```python
from build123d import *

# Parameters (mm, degrees)
SKETCH1_W           = 47.5
SKETCH1_H           = 38.5
SKETCH1_R           = 6.25
SKETCH1_R_2         = 2.75
BOSS_EXTRUDE2_DEPTH = 1
SKETCH2_W           = 61.5
SKETCH2_H           = 44.5
SKETCH2_R           = 1.55
SKETCH2_W_2         = 47.5
SKETCH2_H_2         = 38.5
BOSS_EXTRUDE3_DEPTH = 11.3
SKETCH3_R           = 1.55
BOSS_EXTRUDE4_DEPTH = 2
FILLET2_R           = 4
SKETCH4_W           = 16
SKETCH4_H           = 5.5
CUT_EXTRUDE1_DEPTH  = 8


with BuildPart() as part:
    # Sketch1 → Boss-Extrude2 (new body)
    with BuildSketch(Plane(origin=(0, 0, 0), x_dir=(1, 0, 0), z_dir=(0, 1, 0))):
        Rectangle(SKETCH1_W, SKETCH1_H)
        with Locations(Location((-2.25, 9.8, 0), (0, 0, 270))):
            Circle(SKETCH1_R, mode=Mode.SUBTRACT)
        with Locations(Location((10.75, 0, 0), (0, 0, 270))):
            Circle(SKETCH1_R, mode=Mode.SUBTRACT)
        with Locations(Location((-15.25, 0, 0), (0, 0, 270))):
            Circle(SKETCH1_R, mode=Mode.SUBTRACT)
        with Locations(Location((-2.25, -9.8, 0), (0, 0, 270))):
            Circle(SKETCH1_R, mode=Mode.SUBTRACT)
        with Locations(Location((11.75, 12.05, 0), (0, 0, 270))):
            Circle(SKETCH1_R_2, mode=Mode.SUBTRACT)
    extrude(amount=BOSS_EXTRUDE2_DEPTH)

    # Sketch2 → Boss-Extrude3 (add)
    with BuildSketch(Plane(origin=(0, 1, 0), x_dir=(1, 0, 0), z_dir=(0, 1, 0))):
        Rectangle(SKETCH2_W, SKETCH2_H)
        with Locations(Location((-27.25, 18.75, 0), (0, 0, 270))):
            Circle(SKETCH2_R, mode=Mode.SUBTRACT)
        with Locations(Location((27.25, 18.75, 0), (0, 0, 90))):
            Circle(SKETCH2_R, mode=Mode.SUBTRACT)
        with Locations(Location((27.25, -18.75, 0), (0, 0, 270))):
            Circle(SKETCH2_R, mode=Mode.SUBTRACT)
        with Locations(Location((-27.25, -18.75, 0), (0, 0, 90))):
            Circle(SKETCH2_R, mode=Mode.SUBTRACT)
        Rectangle(SKETCH2_W_2, SKETCH2_H_2, mode=Mode.SUBTRACT)
    extrude(amount=-BOSS_EXTRUDE3_DEPTH)

    # Sketch3 → Boss-Extrude4 (add)
    with BuildSketch(Plane.XZ.offset(-1)):
        with Locations(Location((27.25, -18.75, 0), (0, 0, 270))):
            Circle(SKETCH3_R)
        with Locations(Location((27.25, 18.75, 0), (0, 0, 90))):
            Circle(SKETCH3_R)
        with Locations(Location((-27.25, 18.75, 0), (0, 0, 270))):
            Circle(SKETCH3_R)
        with Locations(Location((-27.25, -18.75, 0), (0, 0, 90))):
            Circle(SKETCH3_R)
    extrude(amount=BOSS_EXTRUDE4_DEPTH)

    # Fillet2
    fillet2_edges = [part.edges().sort_by_distance(p)[0] for p in [
        (-30.75, -4.65, 22.25),
        (-30.75, -4.65, -22.25),
        (30.75, -4.65, -22.25),
        (30.75, -4.65, 22.25),
    ]]
    fillet(fillet2_edges, radius=FILLET2_R)

    # Sketch4 → Cut-Extrude1 (cut)
    with BuildSketch(Plane.ZY.offset(-23.75)):
        with Locations((-5.75, -7.55)):
            Rectangle(SKETCH4_W, SKETCH4_H)
    extrude(amount=-CUT_EXTRUDE1_DEPTH, mode=Mode.SUBTRACT)


solid = part.part
```
Geometry: final body of the model. Coordinates: model frame, mm. A direction names the side the tool comes from. Coordinates: 2 decimals unless noted, no trailing zeros. Loops run counter-clockwise (first coordinate to the right, second up) from the corner with the lowest first, then second, coordinate; pieces in that order, holes last. Notation, with made-up numbers: (22, -8.75) -> (50, -8.75) arc R20 ccw to (50, 2.25) -> close; hole circle Ø4 at (59, -13). An arc over 180 degrees is marked (long way). Use a Markdown table: item, result. Add a question column.
(1) Section query C-C, the plane y = -2.75. Return loops of the section in (x, z), plus the area to 3 significant figures.
(2) Access query for faces 4 (the cylindrical face through (-28.56, -5.58, 17.92)), 5 (the cylindrical face through (-0.37, 0.49, 15.76)). Directions: +Z, -Z, +X, -X, +Y, -Y. A direction counts if a zero-diameter tool reaches every point of the face in a straight line with its end or side. Return the directions, or none.
(3) Section query B-B, the plane z = 9.8. Return loops of the section in (x, y), plus the area to 3 significant figures.
(4) Section query A-A, the plane x = -15.25. Return loops of the section in (y, z), plus the area to 3 significant figures.
(5) Section query D-D, the plane x = -2.25. Return loops of the section in (y, z).
(6) Line query: line 1 along Z through (x, y) = (24, -5.25); line 2 along X through (y, z) = (-8.5, -14.5); line 3 along X through (y, z) = (0.3, 9.8). Output: solid intervals per line, ascending.
(7) Mould query, pull axis Z, two halves, no side actions, for faces 1 (the flat face through (-30.75, -5, 0)), 2 (the cylindrical face through (29.547, -4.729, 21.109)), 3 (the flat face through (23.75, -4, 0)). Classes: pulls with the +Z half, pulls with the -Z half, needs draft (parallel to the pull), parting line crosses it, or undercut.
(8) Pin query (flat end, axial travel): pin 1 Ø6 at (y, z) = (-9, -10.5) entering from +X; pin 2 Ø19 at (x, z) = (8, 2) entering from -Y; pin 3 Ø7.5 at (x, z) = (-2.25, -9.8) entering from +Y; pin 4 Ø2 at (x, z) = (28.5, -5) entering from -Y. Return the tip coordinate at first contact, or that it passes through.
Answer:
| question | item | result |
|---|---|---|
| 1 | outline | (-30.75, -18.25) arc R4 ccw to (-26.75, -22.25) -> (26.75, -22.25) arc R4 ccw to (30.75, -18.25) -> (30.75, 18.25) arc R4 ccw to (26.75, 22.25) -> (-26.75, 22.25) arc R4 ccw to (-30.75, 18.25) -> close; hole circle Ø3.1 at (-27.25, -18.75); hole circle Ø3.1 at (-27.25, 18.75); hole (-23.75, -19.25) -> (23.75, -19.25) -> (23.75, 19.25) -> (-23.75, 19.25) -> close; hole circle Ø3.1 at (27.25, -18.75); hole circle Ø3.1 at (27.25, 18.75) |
| 1 | area | 864 mm^2 |
| 2 | face 4 | -Y |
| 2 | face 5 | +Y, -Y |
| 3 | outline | (-30.75, -10.3) -> (-23.75, -10.3) -> (-23.75, 0) -> (-8.5, 0) -> (-8.5, 1) -> (-30.75, 1) -> close; (4, 0) -> (23.75, 0) -> (23.75, -10.3) -> (30.75, -10.3) -> (30.75, 1) -> (4, 1) -> close |
| 3 | area | 193 mm^2 |
| 4 | outline | (-10.3, -22.25) -> (1, -22.25) -> (1, -6.25) -> (0, -6.25) -> (0, -19.25) -> (-10.3, -19.25) -> close; (-10.3, 19.25) -> (0, 19.25) -> (0, 6.25) -> (1, 6.25) -> (1, 22.25) -> (-10.3, 22.25) -> close |
| 4 | area | 93.8 mm^2 |
| 5 | outline | (-10.3, -22.25) -> (1, -22.25) -> (1, -16.05) -> (0, -16.05) -> (0, -19.25) -> (-10.3, -19.25) -> close; (-10.3, 19.25) -> (0, 19.25) -> (0, 16.05) -> (1, 16.05) -> (1, 22.25) -> (-10.3, 22.25) -> close; (0, -3.55) -> (1, -3.55) -> (1, 3.55) -> (0, 3.55) -> close |
| 6 | line 1 | z = -22.25 to -13.75, 2.25 to 22.25 |
| 6 | line 2 | x = -30.75 to -23.75, 23.75 to 30.75 |
| 6 | line 3 | x = -30.75 to -8.5, 4 to 30.75 |
| 7 | face 1 | needs draft |
| 7 | face 2 | pulls with the +Z half |
| 7 | face 3 | undercut |
| 8 | pin 1 | stops at x = -23.75 |
| 8 | pin 2 | stops at y = 0 |
| 8 | pin 3 | passes through |
| 8 | pin 4 | stops at y = -4.8 |
